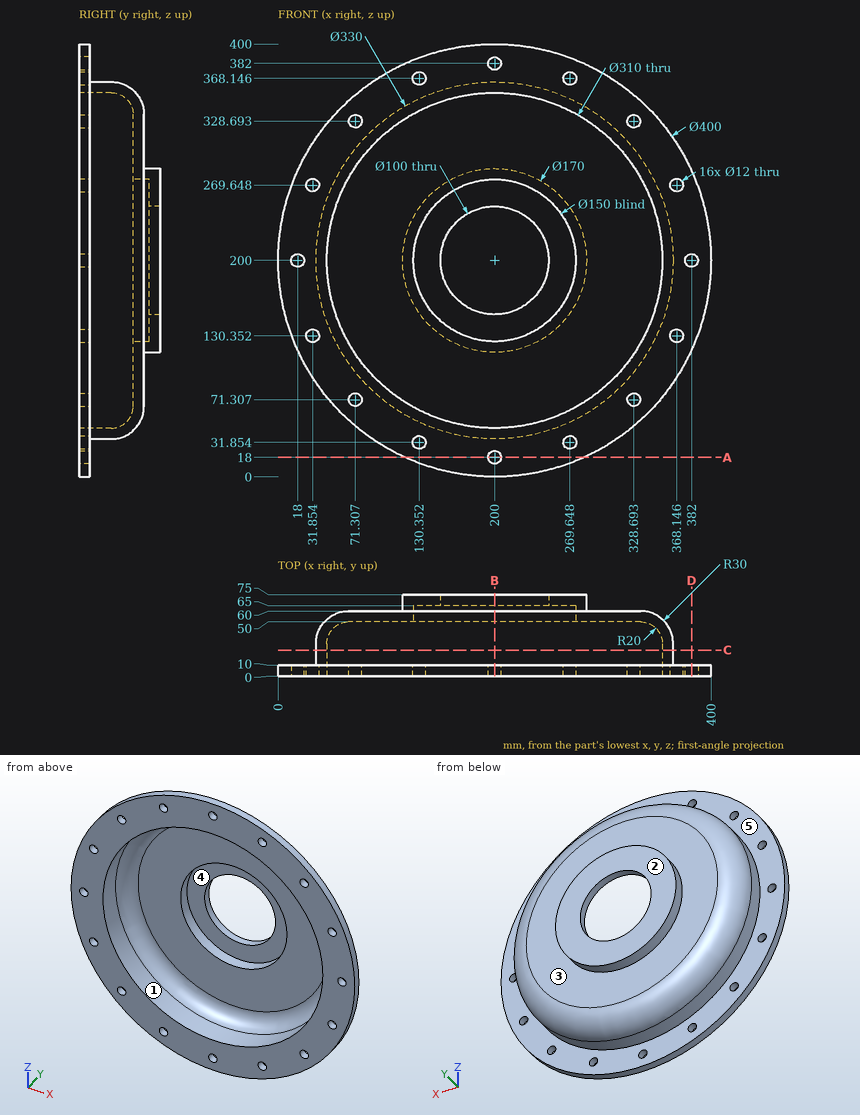
Source: three-view drawing plus pictorial views. Frame: mm from the lowest corner of the part. A direction names the side the tool comes from. Round coordinates to 2 decimals unless told otherwise and drop trailing zeros. Write each loop counter-clockwise with the first axis right and the second up, starting at its lowest first coordinate (ties: lowest second). Pieces come first, ordered by that corner, then holes. Notation, with made-up numbers: (12.5, 12) -> (58.5, 12) arc R27 ccw to (58.5, 43) -> close; hole circle Ø7 at (3, -2.75). An arc over 180 degrees is marked (long way). Return JSON: item names as keys, results as strings.
Q1. Section D-D on x = 382. Return the cut outline in (y, z).
From the geometry:
{"outline": "(0, 117.08) -> (10, 117.08) -> (10, 194) -> (0, 194) -> close; (0, 206) -> (10, 206) -> (10, 282.92) -> (0, 282.92) -> close"}
Q2. First-contact query: pin 1 Ø14 at (x, z) = (328.69, 71.31) entering from +Y; pin 2 Ø5 at (x, y) = (137.5, 33.5) entering from -Z (1 decimal); pin 3 Ø5 at (y, z) = (65, 227) entering from +X; pin 4 Ø7 at (x, z) = (71.31, 328.69) entering from -Y. Flat tips, straight axial feed; report the tip coordinate or a pass-through.
From the geometry:
{"pin 1": "y = 10", "pin 2": "z = 46.5", "pin 3": "x = 281.39", "pin 4": "through"}
Q3. Section C-C on y = 24. Return the cut outline in (x, z).
From the geometry:
{"outline": "circle Ø330 at (200, 200); hole circle Ø310 at (200, 200)"}
Q4. Ray query, line 1 (X direction, y = 4, z = 200); line 2 (Z direction, x = 200, y = 21.5); line 3 (Y direction, x = 175, z = 254). Return the intervals inside material, ascending.
From the geometry:
{"line 1": "0 to 12, 24 to 45, 355 to 376, 388 to 400", "line 2": "35 to 45, 355 to 365", "line 3": "65 to 75"}
Q5. Mould query, pull axis Z, two halves, no side actions, for the marked faces 4 and 5. Classes: +Z half, -Z half, draft (parallel to the pull), parting line (faces both ways), or undercut.
From the geometry:
{"face 4": "undercut", "face 5": "draft"}
Q6. Set-up query: the marked faces 1, 2 and 3. Return all of +Z, -Z, +X, -X, +Y, -Y with unobstructed straight access to the full face (end or side cutting, diameter ignored); none if empty.
From the geometry:
{"face 1": "-Y", "face 2": "+Z, -Z, +X, -X, +Y", "face 3": "+Y"}
Q7. Section B-B on x = 200. Give the number of separate pieces and of enclosed holes in the cut face.
From the geometry:
{"separate pieces": "4", "enclosed holes": "0"}
Q8. Section A-A on z = 18. Return the cut outline in (x, y), and give its area (3 significant figures).
From the geometry:
{"outline": "(117.08, 0) -> (194, 0) -> (194, 10) -> (117.08, 10) -> close; (206, 0) -> (282.92, 0) -> (282.92, 10) -> (206, 10) -> close", "area": "1,540 mm2"}
